from build123d import *

# Parameters (mm, degrees)
SKETCH1_R               = 45
BOSS_EXTRUDE1_DEPTH     = 15
SHELL1_T                = -2
SKETCH11_R              = 43.514084806
BOSS_EXTRUDE4_DEPTH     = 8
SKETCH12_R              = 33
CUT_EXTRUDE2_DEPTH      = 2
SKETCH2_R               = 5
BOSS_EXTRUDE2_DEPTH     = 4.5
SKETCH16_W              = 1.444334904
SKETCH16_H              = 11.111163506
CUT_EXTRUDE3_DEPTH      = 3.5
SKETCH7_R               = 2.4
CUT_EXTRUDE1_DEPTH      = 3.5
SKETCH18_R              = 1.3
CUT_EXTRUDE4_DEPTH      = 17
SKETCH19_R              = 3.5
CUT_EXTRUDE5_DEPTH      = 8
CUT_EXTRUDE6_DEPTH      = 77.485292704
CUT_EXTRUDE6_DEPTH_BACK = 1
SKETCH20_R              = 2
SKETCH22_R              = 20
SKETCH22_R_2            = 12.5
CUT_EXTRUDE10_DEPTH     = 5
CUT_EXTRUDE11_DEPTH     = 6


with BuildPart() as part:
    # Sketch1 → Boss-Extrude1 (new body)
    with BuildSketch(Plane(origin=(0, 0, 0), x_dir=(1, 0, 0), z_dir=(0, 1, 0))):
        with Locations(Location((0, 0, 0), (0, 0, 270))):
            Circle(SKETCH1_R)
    extrude(amount=BOSS_EXTRUDE1_DEPTH)

    # Shell1
    shell1_openings = [part.faces().sort_by_distance(p)[0] for p in [
        (0, 15, 0),
    ]]
    offset(amount=SHELL1_T, openings=shell1_openings, kind=Kind.INTERSECTION)

    # Sketch11 → Boss-Extrude4 (add)
    with BuildSketch(Plane(origin=(0, 2, 0), x_dir=(1, 0, 0), z_dir=(0, 1, 0))):
        with Locations((0, 0.514084806)):
            Circle(SKETCH11_R)
    extrude(amount=BOSS_EXTRUDE4_DEPTH)

    # Sketch12 → Cut-Extrude2 (cut)
    with BuildSketch(Plane(origin=(0, 10, 0), x_dir=(1, 0, 0), z_dir=(0, 1, 0))):
        with Locations(Location((0, 0, 0), (0, 0, 270))):
            Circle(SKETCH12_R)
    extrude(amount=-CUT_EXTRUDE2_DEPTH, mode=Mode.SUBTRACT)

    # Sketch2 → Boss-Extrude2 (add)
    with BuildSketch(Plane(origin=(0, 8, 0), x_dir=(1, 0, 0), z_dir=(0, 1, 0))):
        with Locations(Location((0, 0, 0), (0, 0, 270))):
            Circle(SKETCH2_R)
    extrude(amount=BOSS_EXTRUDE2_DEPTH)

    # Sketch16 → Cut-Extrude3 (cut)
    with BuildSketch(Plane(origin=(0, 12.5, 0), x_dir=(1, 0, 0), z_dir=(0, 1, 0))):
        Rectangle(SKETCH16_W, SKETCH16_H)
    extrude(amount=-CUT_EXTRUDE3_DEPTH, mode=Mode.SUBTRACT)

    # Sketch7 → Cut-Extrude1 (cut)
    with BuildSketch(Plane(origin=(0, 12.5, 0), x_dir=(1, 0, 0), z_dir=(0, 1, 0))):
        Circle(SKETCH7_R)
    extrude(amount=-CUT_EXTRUDE1_DEPTH, mode=Mode.SUBTRACT)

    # Sketch18 → Cut-Extrude4 (cut)
    with BuildSketch(Plane.XZ):
        with Locations(Location((0, 0, 0), (0, 0, 270))):
            Circle(SKETCH18_R)
    extrude(amount=-CUT_EXTRUDE4_DEPTH, mode=Mode.SUBTRACT)

    # Sketch19 → Cut-Extrude5 (cut)
    with BuildSketch(Plane.XZ):
        with Locations(Location((0, 0, 0), (0, 0, 270))):
            Circle(SKETCH19_R)
    extrude(amount=-CUT_EXTRUDE5_DEPTH, mode=Mode.SUBTRACT)

    # Sketch20 → Cut-Extrude6 (cut, two sides: drawn at the far end of the back side and taken through both)
    with BuildSketch(Plane(origin=(15, 0, 0), x_dir=(0, 0, -1), z_dir=(1, 0, 0)).offset(-CUT_EXTRUDE6_DEPTH_BACK)):
        with Locations((-0.169435032, 3)):
            Circle(SKETCH20_R)
    extrude(amount=CUT_EXTRUDE6_DEPTH + CUT_EXTRUDE6_DEPTH_BACK, mode=Mode.SUBTRACT)

    # Sketch22 → Cut-Extrude10 (cut)
    with BuildSketch(Plane(origin=(0, 8, 0), x_dir=(1, 0, 0), z_dir=(0, 1, 0))):
        with Locations(Location((0, 0, 0), (0, 0, 270))):
            Circle(SKETCH22_R)
        with Locations(Location((0, 0, 0), (0, 0, 270))):
            Circle(SKETCH22_R_2, mode=Mode.SUBTRACT)
    extrude(amount=-CUT_EXTRUDE10_DEPTH, mode=Mode.SUBTRACT)

    # Sketch23 → Cut-Extrude11 (cut)
    with BuildSketch(Plane.XZ):
        Polygon((2.862741159, -5.945839979), (6.580619048, -0.493713422), (3.71787789, 5.452126557), (-2.862741159, 5.945839979), (-6.580619048, 0.493713422), (-3.71787789, -5.452126557), align=None)
    extrude(amount=-CUT_EXTRUDE11_DEPTH, mode=Mode.SUBTRACT)


solid = part.part
Read the model definition and answer for the solid it produces. Units are mm, in the model's axes. A direction names the side the tool comes from. Round coordinates to 2 decimals unless told otherwise and drop trailing zeros. Write each loop counter-clockwise with the first axis right and the second up, starting at its lowest first coordinate (ties: lowest second). Pieces come first, ordered by that corner, then holes. Notation, with made-up numbers: (31.5, -28) - (40.5, -28) arc R35 ccw to (40.5, 6) - close; hole circle Ø9 at (56, -28). An arc over 180 degrees is marked (long way). Use a Markdown table: item, result.
(1) The part is cut by section C-C (z = 28.5). Write down the section's boundary in (x, y).
Reported:
| item | result |
|---|---|
| outline | (-34.82, 0) - (34.82, 0) - (34.82, 15) - (32.2, 15) - (32.2, 10) - (16.64, 10) - (16.64, 8) - (-16.64, 8) - (-16.64, 10) - (-32.2, 10) - (-32.2, 15) - (-34.82, 15) - close |
(2) Each of these flat-tipped pins is pushed along its axis until it touches: pin 1 Ø1 at (x, z) = (-9.5, 7.5) entering from +Y; pin 2 Ø6 at (x, y) = (7.5, 4) entering from +Z; pin 3 Ø3 at (y, z) = (11, -4) entering from +X; pin 4 Ø8 at (y, z) = (5, 4) entering from +X. Where does it stop, or does it pass through?
Reported:
| item | result |
|---|---|
| pin 1 | y = 8 |
| pin 2 | z = 44.77 |
| pin 3 | x = 44.93 |
| pin 4 | x = 45 |
(3) The part is cut by section D-D (x = -37.5). Write down the section's boundary in (y, z), then the cut area to 3 significant figures.
Reported:
| item | result |
|---|---|
| outline | (0, -24.87) - (15, -24.87) - (15, -21.04) - (10, -21.04) - (10, 21.04) - (15, 21.04) - (15, 24.87) - (0, 24.87) - close |
| area | 536 mm2 |
(4) The mould has two halves that part along X. Classify faces 4 (the flat face through (-22, 8, 0)), 5 (the cylindrical face through (-17.235, 7.395, 41.569)): released by +X, released by -X, zero draft, split by the parting line, or undercut.
Reported:
| item | result |
|---|---|
| face 4 | undercut |
| face 5 | split by the parting line |
(5) The part is cut by section A-A (x = 28). Write down the section's boundary in (y, z).
Reported:
| item | result |
|---|---|
| outline | (0, -35.23) - (15, -35.23) - (15, -32.63) - (10, -32.63) - (10, -17.46) - (8, -17.46) - (8, 17.46) - (10, 17.46) - (10, 32.63) - (15, 32.63) - (15, 35.23) - (0, 35.23) - close; hole circle Ø4 at (3, 0.17) |
(6) Which of the six approach directions +Z, -Z, +X, -X, +Y, -Y give full straight-line access (tool end or side, diameter ignored) to faces 1 (the cylindrical face through (0.39, 8.49, -1.24)), 2 (the flat face through (-5.17, 2.96, -2.44)), 3 (the flat face through (-0.722, 11, -4))?
Reported:
| item | result |
|---|---|
| face 1 | +Y, -Y |
| face 2 | -Y |
| face 3 | +Y |
(7) The part is cut by section B-B (y = 13.75). Write down the section's boundary in (x, z), then the cut area to 3 significant figures.
Reported:
| item | result |
|---|---|
| outline | circle Ø90 at (0, 0); hole circle Ø86 at (0, 0) |
| area | 553 mm2 |
(8) Straight lines are drawn through the part: line 1 along X through (y, z) = (6.7, 0); line 2 along X through (y, z) = (8.7, 0); line 3 along Z through (x, y) = (8, 7.25). For each, find the intervals that lie inside material, in ascending order. Write a range as [from, to].
Reported:
| item | result |
|---|---|
| line 1 | [-45, -20], [-12.5, -3.5], [3.5, 12.5], [20, 45] |
| line 2 | [-45, -33], [-5, -1.3], [1.3, 5], [33, 45] |
| line 3 | [-44.28, -18.33], [-9.6, 9.6], [18.33, 44.28] |
